The drawing under review shows one solid part. Ordinate dimensions are in mm from its lowest x, y, z. A direction names the side the tool comes from. Round coordinates to 2 decimals unless told otherwise and drop trailing zeros. Order: outer loops, then holes, each group sorted by start corner. A loop starts at its lowest first (then second) coordinate and runs counter-clockwise, first axis right, second up. Notation, with made-up numbers: (23, 67.25) -> (61, 67.25) arc R11 cw to (61, 79.25) -> close; hole circle Ø8 at (72, 31.25). An arc over 180 degrees is marked (long way). Use a Markdown table: item, result. Add a question column.
1) Machinability: for the marked faces 1 and 2, which of the approach directions +Z, -Z, +X, -X, +Y, -Y give a long, thin tool a straight path to every point of the face, cutting with its end or side? Answer none if there is none.
2) Consider section C-C (z = 7.5). State the section outline as (x, y) points.
3) Consider section A-A (y = 13). State the section outline as (x, z) points.
4) Clearance check with flat-ended pins moving along their axes: P1, Ø7, axis at x = 22.5, y = 13.5, coming from the +Z side; P2, Ø2, axis at y = 14.5, z = 7, coming from the -X side. State where each tip first meets the part, or that it passes through.
5) Consider section B-B (x = 14). State the section outline as (y, z) points, plus the area to 3 significant figures.
6) Consider section D-D (x = 23). State the section outline as (y, z) points, plus the area to 3 significant figures.
7) Wall thickness on line 1 along Y through (x, z) = (17, 1.4); line 2 along X through (y, z) = (13, 2.5); line 3 along X through (y, z) = (11, 7): over which ranges is each line inside the solid? List them lowest first. Write a range as [from, to].
8) Draft analysis for pull direction X (two halves, no side actions). For the marked faces 3, 4 and 5, state which applies: pulls with the +X half, pulls with the -X half, needs draft (parallel to the pull), parting line crosses it, or undercut.
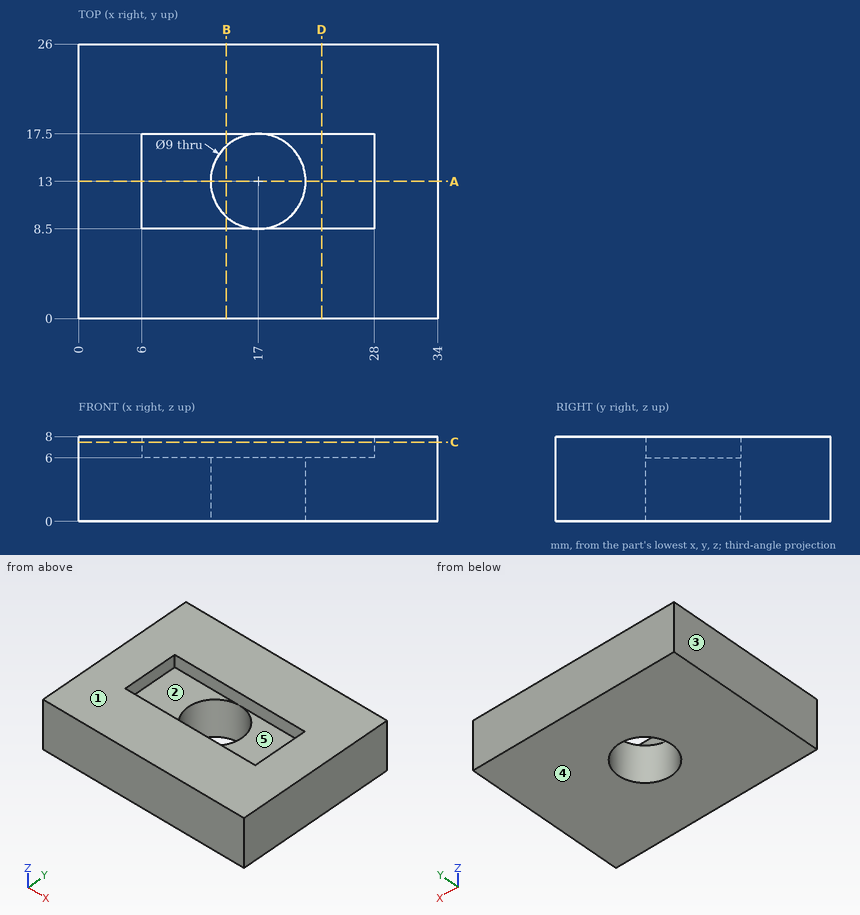
Results list:
| question | item | result |
|---|---|---|
| 1 | face 1 | +Z, +X, -X, +Y, -Y |
| 1 | face 2 | +Z |
| 2 | outline | (0, 0) -> (34, 0) -> (34, 26) -> (0, 26) -> close; hole (6, 8.5) -> (28, 8.5) -> (28, 17.5) -> (6, 17.5) -> close |
| 3 | outline | (0, 0) -> (12.5, 0) -> (12.5, 6) -> (6, 6) -> (6, 8) -> (0, 8) -> close; (21.5, 0) -> (34, 0) -> (34, 8) -> (28, 8) -> (28, 6) -> (21.5, 6) -> close |
| 4 | P1 | z = 6 |
| 4 | P2 | x = 0 |
| 5 | outline | (0, 0) -> (9.65, 0) -> (9.65, 6) -> (8.5, 6) -> (8.5, 8) -> (0, 8) -> close; (16.35, 0) -> (26, 0) -> (26, 8) -> (17.5, 8) -> (17.5, 6) -> (16.35, 6) -> close |
| 5 | area | 150 mm2 |
| 6 | outline | (0, 0) -> (26, 0) -> (26, 8) -> (17.5, 8) -> (17.5, 6) -> (8.5, 6) -> (8.5, 8) -> (0, 8) -> close |
| 6 | area | 190 mm2 |
| 7 | line 1 | [0, 8.5], [17.5, 26] |
| 7 | line 2 | [0, 12.5], [21.5, 34] |
| 7 | line 3 | [0, 6], [28, 34] |
| 8 | face 3 | pulls with the -X half |
| 8 | face 4 | needs draft |
| 8 | face 5 | undercut |
